Work out the finished part from the listing and answer in its coordinate system (mm). A direction names the side the tool comes from. Round coordinates to 2 decimals unless told otherwise and drop trailing zeros. Loops run counter-clockwise (first coordinate to the right, second up) from the corner with the lowest first, then second, coordinate; pieces in that order, holes last.
from build123d import *

# Parameters (mm, degrees)
SKETCH_1_W          = 30
SKETCH_1_H          = 76
EXTRUDE_1_DEPTH     = 2
SKETCH_2_W          = 2
SKETCH_2_H          = 76
EXTRUDE_2_DEPTH     = 30
SKETCH_3_R          = 2.1
CUT_EXTRUDE_3_DEPTH = 88.749643874
SKETCH_4_R          = 1.65
CUT_EXTRUDE_4_DEPTH = 88.749643874


with BuildPart() as part:
    # ｽｹｯﾁ1 → 押し出し1 (new body)
    with BuildSketch(Plane.XY):
        with Locations((15, -38)):
            Rectangle(SKETCH_1_W, SKETCH_1_H)
    extrude(amount=EXTRUDE_1_DEPTH)

    # ｽｹｯﾁ2 → 押し出し2 (add)
    with BuildSketch(Plane.XY.offset(2)):
        with Locations((1, -38)):
            Rectangle(SKETCH_2_W, SKETCH_2_H)
    extrude(amount=EXTRUDE_2_DEPTH)

    # ｽｹｯﾁ3 → 押し出し3 (cut, through all)
    with BuildSketch(Plane(origin=(0, 0, 0), x_dir=(-1, 0, 0), z_dir=(0, 0, -1))):
        with Locations((-27, -4)):
            Circle(SKETCH_3_R)
        with Locations((-27, -72)):
            Circle(SKETCH_3_R)
    extrude(amount=-CUT_EXTRUDE_3_DEPTH, mode=Mode.SUBTRACT)

    # ｽｹｯﾁ4 → 押し出し4 (cut, through all)
    with BuildSketch(Plane.ZY):
        with Locations(Location((6.2, -8, 0), (0, 0, 270))):
            Circle(SKETCH_4_R)
        with Locations(Location((6.2, -24, 0), (0, 0, 270))):
            Circle(SKETCH_4_R)
    extrude(amount=-CUT_EXTRUDE_4_DEPTH, mode=Mode.SUBTRACT)


solid = part.part
Item 1: Determine the mould class of faces 3 (the face through (28.666, -5.278, 0.986)), 4 (the face through (15, -37, 0)), 5 (the face through (1.6, -76, 8.8)), 6 (the face through (1.6, 0, 8.8)) for opening direction Y: pulls with the +Y half, pulls with the -Y half, needs draft (parallel to the pull), parting line crosses it, or undercut.
Item 2: Straight lines are drawn through the part: line 1 (Y direction, x = 27, z = 0.65); line 2 (Z direction, x = 0.9, y = -24); line 3 (Z direction, x = 24.5, y = -8.5). For each, find the intervals that lie inside material, in ascending order.
Item 3: Section C-C, the plane y = -56 is taken. Give the vertices of the cut face in (x, z), plus the area to 3 significant figures.
Item 4: Section A-A, the plane x = 27 is taken. Give the vertices of the cut face in (y, z), plus the area to 3 significant figures.
Item 5: Section B-B, the plane y = -24 is taken. Give the vertices of the cut face in (x, z), plus the area to 3 significant figures.
Item 6: For faces 1 (the face through (0.99, -22.35, 6.27)), 2 (the face through (2, -39, 17)), determine the directions among +Z, -Z, +X, -X, +Y, -Y from which every point of the face is accessible in a straight line to the end or side of a thin tool.
Item 7: Section D-D, the plane x = 20.5 is taken. Give the vertices of the cut face in (y, z).
Item 8: Each of these flat-tipped pins is pushed along its axis until it touches: P1, Ø1.5, axis at x = 5, y = -51.5, coming from the +Z side; P2, Ø9, axis at y = -36, z = 16, coming from the +X side. Where does it stop, or does it pass through?
Answer below:
1. face 3: undercut
1. face 4: needs draft
1. face 5: pulls with the -Y half
1. face 6: pulls with the +Y half
2. line 1: y = -76 to -74.1, -69.9 to -6.1, -1.9 to 0
2. line 2: z = 0 to 4.55, 7.85 to 32
2. line 3: z = 0 to 2
3. outline: (0, 0) - (30, 0) - (30, 2) - (2, 2) - (2, 32) - (0, 32) - close
3. area: 120 mm2
4. outline: (-76, 0) - (-74.1, 0) - (-74.1, 2) - (-76, 2) - close; (-69.9, 0) - (-6.1, 0) - (-6.1, 2) - (-69.9, 2) - close; (-1.9, 0) - (0, 0) - (0, 2) - (-1.9, 2) - close
4. area: 135 mm2
5. outline: (0, 0) - (30, 0) - (30, 2) - (2, 2) - (2, 4.55) - (0, 4.55) - close; (0, 7.85) - (2, 7.85) - (2, 32) - (0, 32) - close
5. area: 113 mm2
6. face 1: +X, -X
6. face 2: +Z, +X, +Y, -Y
7. outline: (-76, 0) - (0, 0) - (0, 2) - (-76, 2) - close
8. P1: stops at z = 2
8. P2: stops at x = 2
